```python
from build123d import *

# Parameters (mm, degrees)
SKETCH1_W           = 42
SKETCH1_H           = 47.5
BOSS_EXTRUDE1_DEPTH = 1
SKETCH2_W           = 5
SKETCH2_H           = 11
SKETCH2_W_2         = 12
SKETCH2_H_2         = 4
CUT_EXTRUDE1_DEPTH  = 5


with BuildPart() as part:
    # Sketch1 → Boss-Extrude1 (new body)
    with BuildSketch(Plane(origin=(0, 0, 0), x_dir=(1, 0, 0), z_dir=(0, 1, 0))):
        Rectangle(SKETCH1_W, SKETCH1_H)
    extrude(amount=BOSS_EXTRUDE1_DEPTH)

    # Sketch2 → Cut-Extrude1 (cut)
    with BuildSketch(Plane(origin=(0, 0, 0), x_dir=(1, 0, 0), z_dir=(0, 1, 0))):
        with Locations((-16.5, 3.25)):
            Rectangle(SKETCH2_W, SKETCH2_H)
        with Locations((0, -18.75)):
            Rectangle(SKETCH2_W_2, SKETCH2_H_2)
    extrude(amount=CUT_EXTRUDE1_DEPTH, mode=Mode.SUBTRACT)


solid = part.part
```
Input: part model. Units: mm. Frame: model coordinates. A direction names the side the tool comes from. Coordinates: 2 decimals unless noted, no trailing zeros. Loops run counter-clockwise (first coordinate to the right, second up) from the corner with the lowest first, then second, coordinate; pieces in that order, holes last. Notation, with made-up numbers: M 29,9 L 69,9 A19 cw 69,21 Z; hole C 9,76.5 d5. An arc over 180 degrees is marked long. Use a Markdown table: item, result. Add a question column.
1) Set-up query: faces 5 (the flat face through (-19, 0.5, -3.2)), 6 (the flat face through (21, 0.5, 0.3)). Return all of +Z, -Z, +X, -X, +Y, -Y with unobstructed straight access to the full face (end or side cutting, diameter ignored); none if empty.
2) Line query: L1, parallel to Z at x = -2, y = 0.3; L2, parallel to X at y = 0.4, z = -8; L3, parallel to Z at x = -14.5, y = 0.95. Output: solid intervals per line, ascending. Write a range as from..to.
3) Section C-C, the plane x = -3.5. Return the cut outline in (y, z), plus the area to 3 significant figures.
4) Draft query along Z for faces 1 (the flat face through (0, 1, 0)), 2 (the flat face through (-0.3, 0.5, 23.75)), 3 (the flat face through (-0.1, 0.5, 16.75)), 4 (the flat face through (-0.3, 0.5, -23.75)). Return one class per face: +Z half, -Z half, draft (parallel to the pull), parting line (faces both ways), or undercut.
5) Section B-B, the plane y = 0.85. Return the cut outline in (x, z).
6) Section A-A, the plane x = -16. Return the cut outline in (y, z), plus the area to 3 significant figures.
Answer below:
| question | item | result |
|---|---|---|
| 1 | face 5 | +Y, -Y |
| 1 | face 6 | +Z, -Z, +X, +Y, -Y |
| 2 | L1 | -23.75..16.75, 20.75..23.75 |
| 2 | L2 | -21..-19, -14..21 |
| 2 | L3 | -23.75..-8.75, 2.25..23.75 |
| 3 | outline | M 0,-23.75 L 1,-23.75 L 1,16.75 L 0,16.75 Z; M 0,20.75 L 1,20.75 L 1,23.75 L 0,23.75 Z |
| 3 | area | 43.5 mm2 |
| 4 | face 1 | draft |
| 4 | face 2 | +Z half |
| 4 | face 3 | undercut |
| 4 | face 4 | -Z half |
| 5 | outline | M -21,-23.75 L 21,-23.75 L 21,23.75 L -21,23.75 Z; hole M -19,-8.75 L -14,-8.75 L -14,2.25 L -19,2.25 Z; hole M -6,16.75 L 6,16.75 L 6,20.75 L -6,20.75 Z |
| 6 | outline | M 0,-23.75 L 1,-23.75 L 1,-8.75 L 0,-8.75 Z; M 0,2.25 L 1,2.25 L 1,23.75 L 0,23.75 Z |
| 6 | area | 36.5 mm2 |
